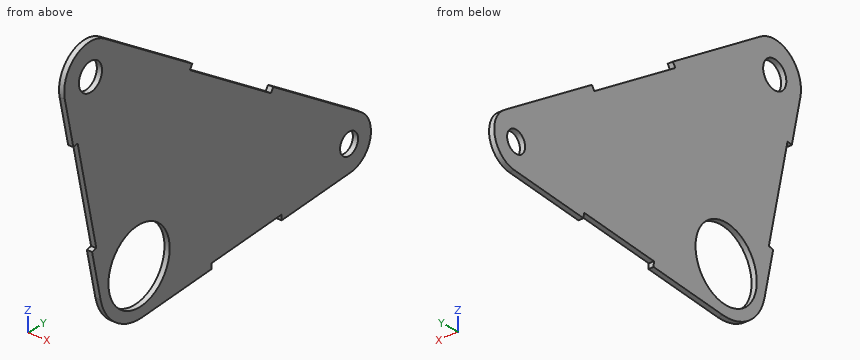
```python
from build123d import *

# Parameters (mm, degrees)
SKETCH1_R               = 11.1125
BOSS_EXTRUDE1_DEPTH     = 1.5875
F_1_4_CLEARANCE_HOLE1_D = 6.5278
M8_CLEARANCE_HOLE1_D    = 8.4


with BuildPart() as part:
    # Sketch1 → Boss-Extrude1 (new body)
    with BuildSketch(Plane(origin=(0, 0, 0), x_dir=(0, 0, -1), z_dir=(1, 0, 0))):
        with BuildLine():
            ThreePointArc((-66.368901101, -12.489303685), (-66.173253482, -23.073465422), (-56.318740763, -26.940161264))
            Line((-56.318740763, -26.940161264), (-42.141879325, -23.840144889))
            Line((-42.141879325, -23.840144889), (-42.481000758, -22.28928935))
            Line((-42.481000758, -22.28928935), (-11.463889973, -15.506860689))
            Line((-11.463889973, -15.506860689), (-11.12476854, -17.057716228))
            Line((-11.12476854, -17.057716228), (3.052092897, -13.957699853))
            ThreePointArc((3.052092897, -13.957699853), (11.493610044, -8.487024473), (14.237804197, 1.190625))
            Line((14.237804197, 1.190625), (12.135875062, 26.326041667))
            Line((12.135875062, 26.326041667), (10.553896818, 26.19375))
            Line((10.553896818, 26.19375), (8.429842112, 51.59375))
            Line((8.429842112, 51.59375), (10.011820356, 51.726041667))
            Line((10.011820356, 51.726041667), (7.909891221, 76.861458333))
            ThreePointArc((7.909891221, 76.861458333), (1.914833772, 83.903071977), (-6.67952645, 80.488103619))
            Line((-6.67952645, 80.488103619), (-27.090385813, 48.694358158))
            Line((-27.090385813, 48.694358158), (-25.754480523, 47.836737434))
            Line((-25.754480523, 47.836737434), (-44.622136448, 18.446821053))
            Line((-44.622136448, 18.446821053), (-45.958041738, 19.304441777))
            Line((-45.958041738, 19.304441777), (-66.368901101, -12.489303685))
        make_face()
        Circle(SKETCH1_R, mode=Mode.SUBTRACT)
    extrude(amount=BOSS_EXTRUDE1_DEPTH)

    # 1/4 Clearance Hole1 (through all)
    with Locations(Plane(origin=(1.5875, 0, 0), x_dir=(0, 0, -1), z_dir=(1, 0, 0))):
        with Locations((0, 76.2)):
            Hole(F_1_4_CLEARANCE_HOLE1_D / 2)

    # M8 Clearance Hole1 (through all)
    with Locations(Plane(origin=(1.5875, 0, 0), x_dir=(0, 0, -1), z_dir=(1, 0, 0))):
        with Locations((-58.353469361, -17.635028028)):
            Hole(M8_CLEARANCE_HOLE1_D / 2)


solid = part.part
```
The model under review builds one solid part; all positions refer to its coordinate system, in mm. Coordinates: 2 decimals unless noted, no trailing zeros. Order: outer loops, then holes, each group sorted by start corner. A loop starts at its lowest first (then second) coordinate and runs counter-clockwise, first axis right, second up. Notation, with made-up numbers: (-11.5, 31.5) -> (41.5, 31.5) arc R10 cw to (41.5, 48.5) -> close; hole circle Ø1 at (78.5, 63). An arc over 180 degrees is marked (long way). Answer in a Markdown table with one row per item. Add a question column.
Item 1: We need section D-D on z = 15. Write out the cut boundary in (x, y).
Item 2: We need section A-A on x = 0.7. Give the number of separate pieces and of enclosed holes in the cut face, plus the area to 3 significant figures.
Item 3: To check wall thickness, follow probe 1 along Y at (x, z) = (0.85, 0); probe 2 along Y at (x, z) = (1.1, 60); probe 3 along Y at (x, z) = (1.25, 61). State the ranges of each line that lie inside material, in increasing order.
Item 4: We need section C-C on y = 16. Write out the cut boundary in (x, z).
Item 5: Clearance check with a flat-ended pin moving along its axis: pin 1 (7.5 mm diameter, centred on y = 76.2, z = 0, fed in from -X). State where the tip first meets the part, or that it passes through.
Item 6: We need section B-B on z = 61. Write out the cut boundary in (x, y), plus the area to 3 significant figures.
Final values:
| question | item | result |
|---|---|---|
| 1 | outline | (0, -16.28) -> (1.59, -16.28) -> (1.59, 67.53) -> (0, 67.53) -> close |
| 2 | separate pieces | 1 |
| 2 | enclosed holes | 3 |
| 2 | area | 4,460 mm2 |
| 3 | probe 1 | y = -14.63 to -11.11, 11.11 to 72.94, 79.46 to 84.14 |
| 3 | probe 2 | y = -27.02 to -21.5, -13.77 to -2.57 |
| 3 | probe 3 | y = -26.78 to -20.9, -14.37 to -4.13 |
| 4 | outline | (0, -13) -> (1.59, -13) -> (1.59, 48.08) -> (0, 48.08) -> close |
| 5 | pin 1 | stops at x = 0 |
| 6 | outline | (0, -26.78) -> (1.59, -26.78) -> (1.59, -20.9) -> (0, -20.9) -> close; (0, -14.37) -> (1.59, -14.37) -> (1.59, -4.13) -> (0, -4.13) -> close |
| 6 | area | 25.6 mm2 |
